```python
from build123d import *

# Parameters (mm, degrees)
F1_DEPTH = 44.45
F3_R     = 5.08


# Not quite as in the source:
# - a feature of the source that left no trace in its solid (it failed there, or was rolled back) is left out


with BuildPart() as f1:
    # F0 (on Right) → F1 (new body, symmetric)
    with BuildSketch(Plane.YZ):
        Polygon((19.6727830917, 30.9194792062), (-33.4437340498, 30.9194792062), (-33.4437340498, -13.377064839), (19.6727830917, -18.1674808264), align=None)
    extrude(amount=F1_DEPTH, both=True)

    # F3
    f3_edges = [f1.edges().sort_by_distance(p)[0] for p in [
        (-44.45, 19.672783, 6.375999),
        (-44.45, -6.885475, 30.919479),
        (0, -33.443734, 30.919479),
        (44.45, -6.885475, 30.919479),
        (0, 19.672783, 30.919479),
        (44.45, 19.672783, 6.375999),
        (0, 19.672783, -18.167481),
        (0, -33.443734, -13.377065),
        (-44.45, -6.885475, -15.772273),
        (44.45, -6.885475, -15.772273),
        (44.45, -33.443734, 8.771207),
        (-44.45, -33.443734, 8.771207),
    ]]
    fillet(f3_edges, radius=F3_R)


solid = f1.part
```
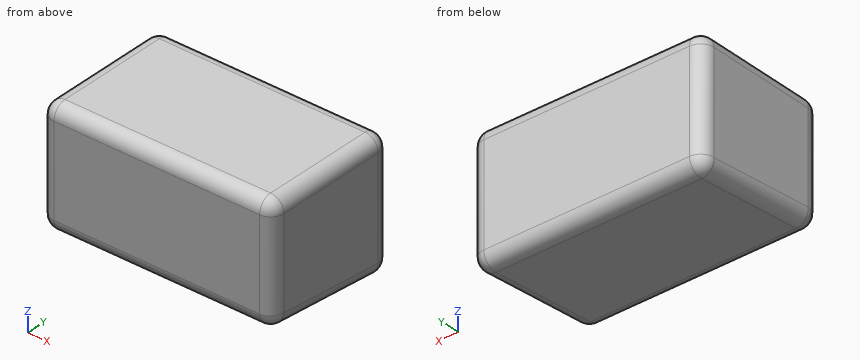
Source: CAD feature listing. Evaluate the final solid. Frame: model axes, mm. Coordinates: 2 decimals unless noted, no trailing zeros. Loops run counter-clockwise (first coordinate to the right, second up) from the corner with the lowest first, then second, coordinate; pieces in that order, holes last. Notation, with made-up numbers: M 82,43.5 L 114,43.5 A15 cw 114,48.5 Z; hole C 2,58.5 d4. An arc over 180 degrees is marked long. Use a Markdown table: item, result. Add a question column.
Q1. Section query B-B, the plane z = 28. Return loops of the section in (x, y).
Q2. Section query A-A, the plane x = -35.5. Return loops of the section in (y, z), and give its area (3 significant figures).
Q3. First-contact query: pin 1 (10 mm diameter, centred on x = 15.5, y = -3, fed in from -Z); pin 2 (2 mm diameter, centred on x = 26.5, y = -7, fed in from -Z). Flat tips, straight axial feed; report the tip coordinate or a pass-through.
Q4. Material intervals for L1, parallel to Z at x = 21, y = -1; L2, parallel to Z at x = 34, y = -28; L3, parallel to Y at x = -27.5, z = -12.5, sorted ascending.
Result:
| question | item | result |
|---|---|---|
| 1 | outline | M -43.97,-28.36 A4.6 ccw -39.37,-32.96 L 39.37,-32.96 A4.6 ccw 43.97,-28.36 L 43.97,14.59 A4.6 ccw 39.37,19.19 L -39.37,19.19 A4.6 ccw -43.97,14.59 Z |
| 2 | outline | M -33.44,-8.73 A5.08 ccw -28.82,-13.79 L 14.14,-17.67 A5.08 ccw 19.67,-12.61 L 19.67,25.84 A5.08 ccw 14.59,30.92 L -28.36,30.92 A5.08 ccw -33.44,25.84 Z |
| 2 | area | 2,460 mm2 |
| 3 | pin 1 | stops at z = -16.57 |
| 3 | pin 2 | stops at z = -15.85 |
| 4 | L1 | z = -16.3 to 30.92 |
| 4 | L2 | z = -13.87 to 30.92 |
| 4 | L3 | y = -31.77 to 19.67 |
